```python
from build123d import *

# Parameters (mm, degrees)
F0_W     = 164.7579842525
F0_H     = 120
F1_DEPTH = 5
F2_W     = 31.3406437635
F2_H     = 119.9177950621
F3_DEPTH = 29.5
F4_W     = 119.9177950621
F4_H     = 0.25
F5_DEPTH = 15
F6_W     = 0.25
F6_H     = 110
F7_DEPTH = 22.76


with BuildPart() as f1:
    # F0 (on Top) → F1 (new body)
    with BuildSketch(Plane.XY):
        Rectangle(F0_W, F0_H)
    extrude(amount=F1_DEPTH)

    # F2 (on Top) → F3 (join)
    with BuildSketch(Plane.XY):
        with Locations((66.5988624096, 0)):
            Rectangle(F2_W, F2_H)
    extrude(amount=F3_DEPTH)

    # F4 (on face) → F5 (cut)
    with BuildSketch(Plane(origin=(50.9285405278, 0, 0), x_dir=(0, -1, 0), z_dir=(-1, 0, 0))):
        with Locations((0, 6.625)):
            Rectangle(F4_W, F4_H)
    extrude(amount=-F5_DEPTH, mode=Mode.SUBTRACT)

    # F6 (on face) → F7 (cut)
    with BuildSketch(Plane.XY.offset(29.5)):
        with Locations((66.5988624096, 0)):
            Rectangle(F6_W, F6_H)
    extrude(amount=-F7_DEPTH, mode=Mode.SUBTRACT)


solid = f1.part
```
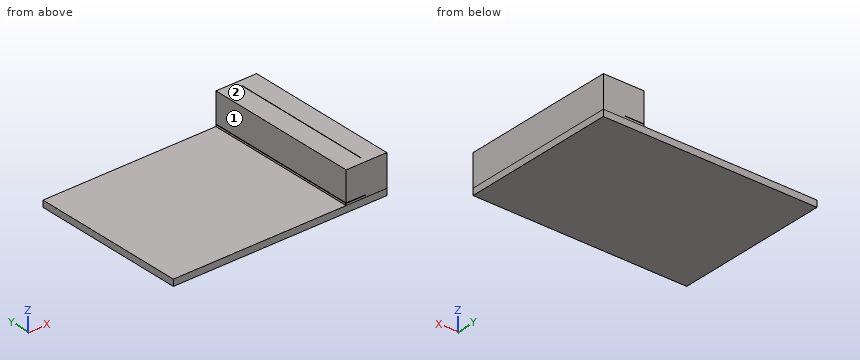
The model under review builds one solid part; all positions refer to its coordinate system, in mm. Face numbers are marked on the shaded views. A direction names the side the tool comes from. Give positions to 0.01 mm unless a question says otherwise; leave off trailing zeros. Write each loop counter-clockwise with the first axis right and the second up, starting at its lowest first coordinate (ties: lowest second). Pieces come first, ordered by that corner, then holes.
(1) Consider section C-C, the plane x = -33. Give the boundary of the cut face in (y, z).
(2) To check wall thickness, follow L1, parallel to X at y = -15, z = 15; L2, parallel to Z at x = 59.5, y = -5.5; L3, parallel to Z at x = 8.5, y = -39. State the ranges of each line that lie inside material, in increasing order.
(3) Consider section A-A, the plane z = 17.25. Give the boundary of the cut face in (x, y).
(4) Tool access review of the marked faces 1 and 2: name each direction out of +Z, -Z, +X, -X, +Y, -Y from which nothing blocks a thin tool from reaching the whole face with its end or side.
(5) Consider section B-B, the plane y = -29. Give the boundary of the cut face in (x, z).
(6) For P1, Ø1, axis at y = -43.5, z = 19.5, coming from the -X side; P2, Ø8, axis at x = -4.5, y = -9.5, coming from the +Z side; P3, Ø7.5, axis at y = -13.5, z = 15.5, coming from the +X side, all flat-tipped, find the tip position at first contact; note any pin that passes through.
Returned:
1. outline: (-60, 0) - (60, 0) - (60, 5) - (-60, 5) - close
2. L1: x = 50.93 to 66.47, 66.72 to 82.27
2. L2: z = 0 to 6.5, 6.75 to 29.5
2. L3: z = 0 to 5
3. outline: (50.93, -59.96) - (82.27, -59.96) - (82.27, 59.96) - (50.93, 59.96) - close; hole (66.47, -55) - (66.72, -55) - (66.72, 55) - (66.47, 55) - close
4. face 1: +Z, -X, +Y, -Y
4. face 2: +Z, +X, -X, +Y, -Y
5. outline: (-82.38, 0) - (82.38, 0) - (82.38, 5) - (82.27, 5) - (82.27, 29.5) - (66.72, 29.5) - (66.72, 6.74) - (66.47, 6.74) - (66.47, 29.5) - (50.93, 29.5) - (50.93, 6.75) - (65.93, 6.75) - (65.93, 6.5) - (50.93, 6.5) - (50.93, 5) - (-82.38, 5) - close
6. P1: stops at x = 50.93
6. P2: stops at z = 5
6. P3: stops at x = 82.27
